```python
from build123d import *

# Parameters (mm, degrees)
F1_DEPTH = 42
F2_W     = 16
F2_H     = 25
F3_DEPTH = 10
F4_W     = 25
F4_H     = 9
F5_DEPTH = 16.001


with BuildPart() as f1:
    # F0 (on Front) → F1 (new body)
    with BuildSketch(Plane.XZ):
        Polygon((0, 42), (0, 0), (58, 0), (58, 16), (16, 16), (16, 42), align=None)
    extrude(amount=F1_DEPTH)

    # F2 (on face) → F3 (cut)
    with BuildSketch(Plane.XY.offset(42)):
        with Locations((8, -20.5)):
            Rectangle(F2_W, F2_H)
    extrude(amount=-F3_DEPTH, mode=Mode.SUBTRACT)

    # F4 (on face) → F5 (cut, through all)
    with BuildSketch(Plane.XY.offset(16)):
        with Locations((45.5, -21.5)):
            Rectangle(F4_W, F4_H)
    extrude(amount=-F5_DEPTH, mode=Mode.SUBTRACT)


solid = f1.part
```
Source: CAD feature listing. Evaluate the final solid. Frame: model axes, mm. A direction names the side the tool comes from. Round coordinates to 2 decimals unless told otherwise and drop trailing zeros. Write each loop counter-clockwise with the first axis right and the second up, starting at its lowest first coordinate (ties: lowest second). Pieces come first, ordered by that corner, then holes. Notation, with made-up numbers: M 69,82 L 113,82 A20 cw 113,90 Z; hole C -30.5,-32 d2. An arc over 180 degrees is marked long. Answer as a JSON object with one key per item and string values. Group by question number.
(1) Section query C-C on x = 4.5. Output: boundary loops of the cut face in (y, z), then the cut area to 3 significant figures.
(2) Section query A-A on x = 37.5. Output: boundary loops of the cut face in (y, z).
(3) Section query D-D on y = -24.5. Output: boundary loops of the cut face in (x, z).
(4) Section query B-B on z = 8.5. Output: boundary loops of the cut face in (x, y), then the cut area to 3 significant figures.
(5) First-contact query: pin 1 (5 mm diameter, centred on x = 7, y = -23.5, fed in from +Z); pin 2 (13 mm diameter, centred on y = -20.5, z = 28, fed in from +X). Flat tips, straight axial feed; report the tip coordinate or a pass-through.
(6) Reachability of faces 1 (the flat face through (45, -17, 8)), 2 (the flat face through (32.6, -20.7, 16)), 3 (the flat face through (8, -20, 32)) from +Z, -Z, +X, -X, +Y, -Y: full face, straight path, thin tool, end or side. Return the list, or none.
(7) Ray query, line 1 (Y direction, x = 13.5, z = 40.5); line 2 (Y direction, x = 45, z = 10); line 3 (Z direction, x = 36, y = -9). Return the intervals inside material, ascending. Write a range as [from, to].
(8) Mould query, pull axis Y, two halves, no side actions, for faces 4 (the flat face through (0, -21, 21)), 5 (the flat face through (33, -22, 8)), 6 (the flat face through (22, 0, 12)). Classes: +Y half, -Y half, draft (parallel to the pull), parting line (faces both ways), or undercut.
Computed values:
{
 "1": {"outline": "M -42,0 L 0,0 L 0,42 L -8,42 L -8,32 L -33,32 L -33,42 L -42,42 Z", "area": "1,510 mm^2"},
 "2": {"outline": "M -42,0 L -26,0 L -26,16 L -42,16 Z; M -17,0 L 0,0 L 0,16 L -17,16 Z"},
 "3": {"outline": "M 0,0 L 33,0 L 33,16 L 16,16 L 16,32 L 0,32 Z"},
 "4": {"outline": "M 0,-42 L 58,-42 L 58,-26 L 33,-26 L 33,-17 L 58,-17 L 58,0 L 0,0 Z", "area": "2,210 mm^2"},
 "5": {"pin 1": "z = 32", "pin 2": "x = 16"},
 "6": {"face 1": "+Z, -Z, +X", "face 2": "+Z, +X, +Y, -Y", "face 3": "+Z, +X, -X"},
 "7": {"line 1": "[-42, -33], [-8, 0]", "line 2": "[-42, -26], [-17, 0]", "line 3": "[0, 16]"},
 "8": {"face 4": "draft", "face 5": "undercut", "face 6": "+Y half"}
}
